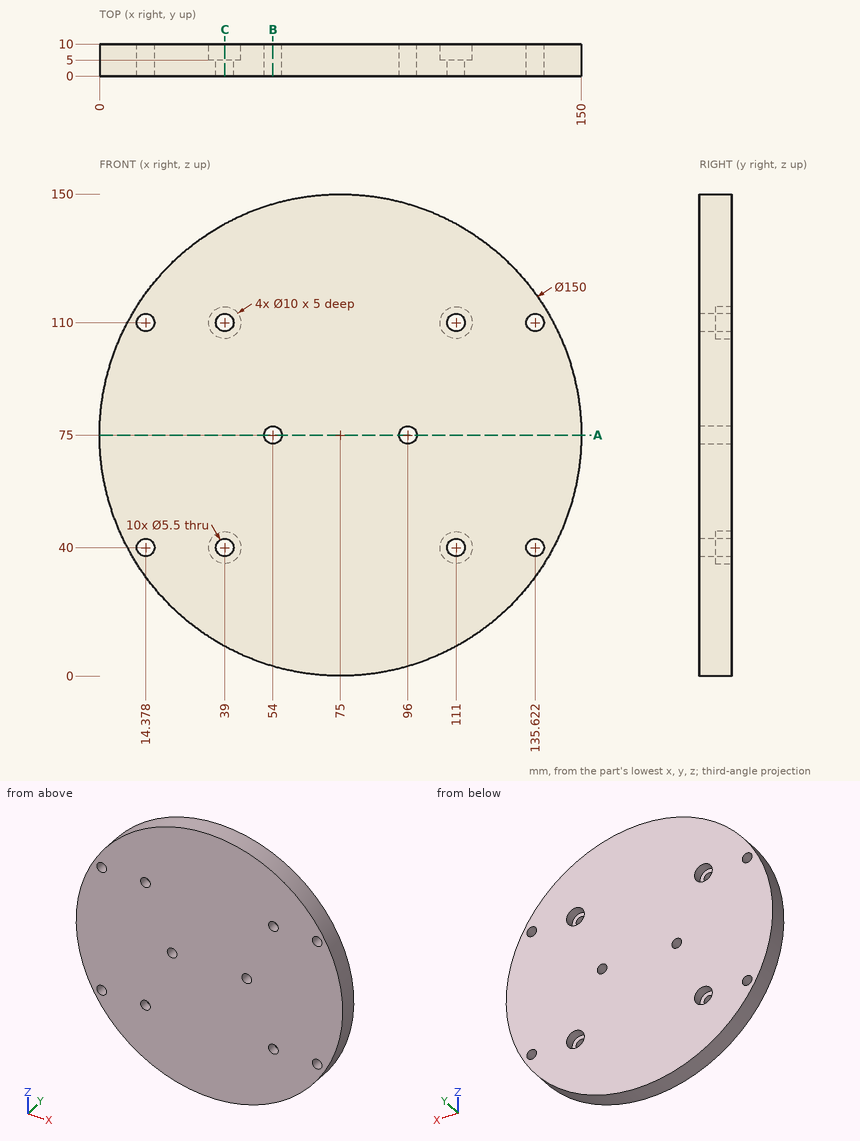
For this review, use the dimensioned drawing (mm, ordinates from the lowest corner) and the shaded views. Round coordinates to 2 decimals unless told otherwise and drop trailing zeros. Order: outer loops, then holes, each group sorted by start corner. A loop starts at its lowest first (then second) coordinate and runs counter-clockwise, first axis right, second up. Notation, with made-up numbers: M 26.5,72.5 L 84.5,72.5 A24 cw 84.5,85.5 Z; hole C 21,-23 d10. An arc over 180 degrees is marked long. Use a Markdown table: item, result.
1) Wall thickness on line 1 along X through (y, z) = (6.25, 75); line 2 along X through (y, z) = (3.5, 39) (1 decimal); line 3 along X through (y, z) = (3.5, 110): over which ranges is each line inside the solid? List them lowest first. Write a range as [from, to].
Report:
| item | result |
|---|---|
| line 1 | [0, 51.25], [56.75, 93.25], [98.75, 150] |
| line 2 | [9.2, 11.8], [16.9, 36.4], [41.6, 108.4], [113.6, 133.1], [138.2, 140.8] |
| line 3 | [8.67, 11.63], [17.13, 36.25], [41.75, 108.25], [113.75, 132.87], [138.37, 141.33] |
2) Consider section A-A (z = 75). Write out the cut boundary in (x, y).
Report:
| item | result |
|---|---|
| outline | M 0,0 L 51.25,0 L 51.25,10 L 0,10 Z; M 56.75,0 L 93.25,0 L 93.25,10 L 56.75,10 Z; M 98.75,0 L 150,0 L 150,10 L 98.75,10 Z |
3) Consider section C-C (x = 39). Give the number of separate pieces and of enclosed holes in the cut face, then the cut area to 3 significant figures.
Report:
| item | result |
|---|---|
| separate pieces | 3 |
| enclosed holes | 0 |
| area | 1,160 mm^2 |
4) Insertion check: pin 1 (7 mm diameter, centred on x = 39, z = 110, fed in from +Y); pin 2 (2 mm diameter, centred on x = 129, y = 1, fed in from -Z); pin 3 (3 mm diameter, centred on y = 1.5, z = 23, fed in from +X). Each pin has a flat end and moves straight along its axis. Give the tip position at first contact, or say it passes through.
Report:
| item | result |
|---|---|
| pin 1 | y = 5 |
| pin 2 | z = 21.93 |
| pin 3 | x = 130.45 |
5) Consider section B-B (x = 54). Write out the cut boundary in (y, z).
Report:
| item | result |
|---|---|
| outline | M 0,3 L 10,3 L 10,72.25 L 0,72.25 Z; M 0,77.75 L 10,77.75 L 10,147 L 0,147 Z |
